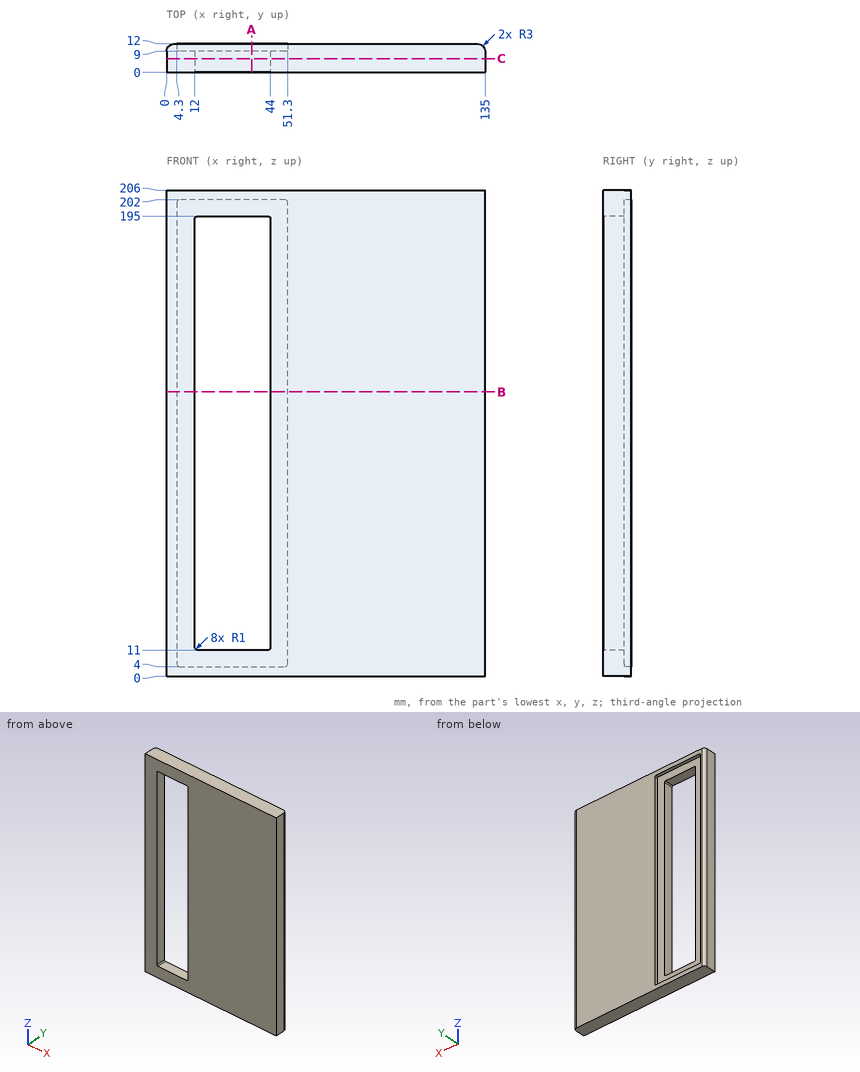
Check sheet for the drawn part. Datum: minimum x, y, z corner. Units: mm. Round coordinates to 2 decimals unless told otherwise and drop trailing zeros. Loops run counter-clockwise (first coordinate to the right, second up) from the corner with the lowest first, then second, coordinate; pieces in that order, holes last. Notation, with made-up numbers: M 40,85 L 91,85 A33 ccw 91,118 Z; hole C 41,50 d9. An arc over 180 degrees is marked long. One line per question, with ' | ' between items. Start each with the question number.
Item 1: Gauge pin test, flat ends, axial feed: pin 1 Ø0.9 at (y, z) = (10.5, 75.5) entering from +X; pin 2 Ø0.9 at (y, z) = (10, 75) entering from -X. Record the tip position at first contact, or that the pin passes through.
Item 2: Scan lines: probe 1 along X at (y, z) = (8, 134); probe 2 along Z at (x, y) = (35, 7.75); probe 3 along X at (y, z) = (9.5, 97). Record each from-to range of solid material in increasing order.
Item 3: Section check B-B (z = 120.5). Record the boundary of the cut face in (x, y).
Item 4: Section check A-A (x = 36). Record the boundary of the cut face in (y, z).
Item 5: Section check C-C (y = 5.75). Record the boundary of the cut face in (x, z), and give its area (3 significant figures).
Worked out:
1) pin 1: x = 134.81 | pin 2: x = 0.05
2) probe 1: 0 to 12, 44 to 135 | probe 2: 0 to 11, 195 to 206 | probe 3: 0.04 to 4.3, 51.3 to 134.96
3) outline: M 0,0 L 12,0 L 12,9 L 4.3,9 L 4.3,12 L 3,12 A3 ccw 0,9 Z; M 44,0 L 135,0 L 135,9 A3 ccw 132,12 L 51.3,12 L 51.3,9 L 44,9 Z
4) outline: M 0,0 L 12,0 L 12,4 L 9,4 L 9,11 L 0,11 Z; M 0,195 L 9,195 L 9,202 L 12,202 L 12,206 L 0,206 Z
5) outline: M 0,0 L 135,0 L 135,206 L 0,206 Z; hole M 12,12 A1 ccw 13,11 L 43,11 A1 ccw 44,12 L 44,194 A1 ccw 43,195 L 13,195 A1 ccw 12,194 Z | area: 21,900 mm^2
